```python
from build123d import *

# Parameters (mm, degrees)
F0_W     = 15
F0_H     = 25
F0_W_2   = 11
F0_H_2   = 21
F1_DEPTH = 2.4
F2_W     = 18
F2_H     = 28
F2_W_2   = 15
F2_H_2   = 25
F2_W_3   = 11
F2_H_3   = 21
F3_DEPTH = 1.5
F4_W     = 4.5
F4_H     = 2
F4_W_2   = 2
F4_H_2   = 9.5
F5_DEPTH = 3.9


with BuildPart() as f1:
    # F0 (on Front) → F1 (new body)
    with BuildSketch(Plane.XZ):
        Rectangle(F0_W, F0_H)
        Rectangle(F0_W_2, F0_H_2, mode=Mode.SUBTRACT)
    extrude(amount=F1_DEPTH)

    # F2 (on face) → F3 (join)
    with BuildSketch(Plane.XZ.offset(2.4)):
        Rectangle(F2_W, F2_H)
        Rectangle(F2_W_2, F2_H_2, mode=Mode.SUBTRACT)
        Rectangle(F2_W_2, F2_H_2)
        Rectangle(F2_W_3, F2_H_3, mode=Mode.SUBTRACT)
    extrude(amount=F3_DEPTH)

    # F4 (on face) → F5 (join)
    with BuildSketch(Plane.XZ.offset(3.9)):
        with Locations((-3.25, 0)):
            Rectangle(F4_W, F4_H)
        with Locations((0, 5.75)):
            Rectangle(F4_W_2, F4_H_2)
        Rectangle(F4_W_2, F4_H)
        with Locations((3.25, 0)):
            Rectangle(F4_W, F4_H)
        with Locations((0, -5.75)):
            Rectangle(F4_W_2, F4_H_2)
    extrude(amount=-F5_DEPTH)


solid = f1.part
```
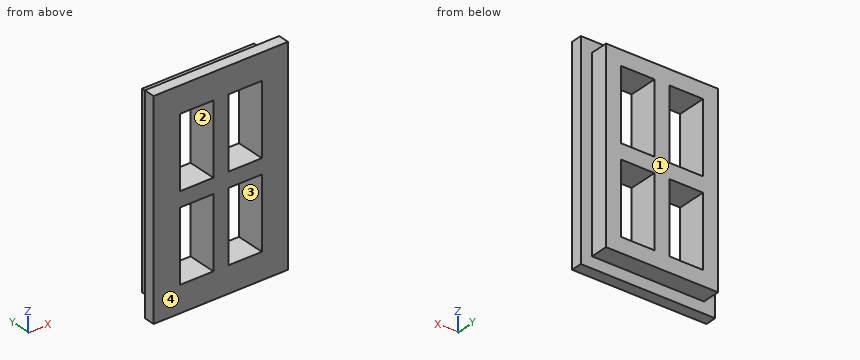
Geometry: final body of the model. Coordinates: model frame, mm. Face numbers are marked on the shaded views. A direction names the side the tool comes from. Round coordinates to 2 decimals unless told otherwise and drop trailing zeros. Write each loop counter-clockwise with the first axis right and the second up, starting at its lowest first coordinate (ties: lowest second). Pieces come first, ordered by that corner, then holes.
Item 1: Set-up query: the marked faces 3 and 4. Return all of +Z, -Z, +X, -X, +Y, -Y with unobstructed straight access to the full face (end or side cutting, diameter ignored); none if empty.
Item 2: Section query D-D (y = -0.3). Return loops of the section in (x, z), plus the area to 3 significant figures.
Item 3: Section query C-C (x = -7). Return loops of the section in (y, z), plus the area to 3 significant figures.
Item 4: Section query A-A (x = 3.5). Return loops of the section in (y, z).
Item 5: Material intervals for L1, parallel to Z at x = -4, y = -0.15; L2, parallel to X at y = -1.3, z = -8; L3, parallel to X at y = -3.2, z = 4.5, sorted ascending.
Item 6: Section query B-B (z = 11.75). Return loops of the section in (x, y), plus the area to 3 significant figures.
Item 7: Mould query, pull axis Z, two halves, no side actions, for the marked faces 1 and 2. Classes: +Z half, -Z half, draft (parallel to the pull), parting line (faces both ways), or undercut.
Item 8: Pin query (flat end, axial travel): P1, Ø1.2, axis at x = -3, y = -1.5, coming from the +Z side; P2, Ø1.2, axis at y = -1.5, z = 1, coming from the +X side; P3, Ø0.7, axis at x = 2.5, y = -0.5, coming from the -Z side. Return the tip coordinate at first contact, or that it passes through.
Completed:
1. face 3: +Y, -Y
1. face 4: +Z, -Z, +X, -X, -Y
2. outline: (-7.5, -12.5) - (7.5, -12.5) - (7.5, 12.5) - (-7.5, 12.5) - close; hole (-5.5, -10.5) - (-1, -10.5) - (-1, -1) - (-5.5, -1) - close; hole (-5.5, 1) - (-1, 1) - (-1, 10.5) - (-5.5, 10.5) - close; hole (1, -10.5) - (5.5, -10.5) - (5.5, -1) - (1, -1) - close; hole (1, 1) - (5.5, 1) - (5.5, 10.5) - (1, 10.5) - close
2. area: 204 mm2
3. outline: (-3.9, -14) - (-2.4, -14) - (-2.4, -12.5) - (0, -12.5) - (0, 12.5) - (-2.4, 12.5) - (-2.4, 14) - (-3.9, 14) - close
3. area: 102 mm2
4. outline: (-3.9, -14) - (-2.4, -14) - (-2.4, -12.5) - (0, -12.5) - (0, -10.5) - (-3.9, -10.5) - close; (-3.9, -1) - (0, -1) - (0, 1) - (-3.9, 1) - close; (-3.9, 10.5) - (0, 10.5) - (0, 12.5) - (-2.4, 12.5) - (-2.4, 14) - (-3.9, 14) - close
5. L1: z = -12.5 to -10.5, -1 to 1, 10.5 to 12.5
5. L2: x = -7.5 to -5.5, -1 to 1, 5.5 to 7.5
5. L3: x = -9 to -5.5, -1 to 1, 5.5 to 9
6. outline: (-9, -3.9) - (9, -3.9) - (9, -2.4) - (7.5, -2.4) - (7.5, 0) - (-7.5, 0) - (-7.5, -2.4) - (-9, -2.4) - close
6. area: 63.0 mm2
7. face 1: draft
7. face 2: undercut
8. P1: stops at z = 12.5
8. P2: stops at x = 7.5
8. P3: stops at z = -12.5
